Can you work these out from the drawing? Everything is in mm from the part's minimum corner. A direction names the side the tool comes from. Round coordinates to 2 decimals unless told otherwise and drop trailing zeros. Order: outer loops, then holes, each group sorted by start corner. A loop starts at its lowest first (then second) coordinate and runs counter-clockwise, first axis right, second up. Notation, with made-up numbers: M 38.25,47 L 89.25,47 A27 ccw 89.25,75 Z; hole C -30,39.5 d7. An arc over 180 degrees is marked long. Write item = value, one per line. Start each with the question number.
Item 1: For the marked faces 4 and 5, which set-ups out of +Z, -Z, +X, -X, +Y, -Y let a thin tool reach every point of the face, with its end or its side?
Item 2: I want a section at C-C, the plane z = 4.75. List the corners of the cut face in (x, y) for me (3 decimals), plus the area to 3 significant figures.
Item 3: I want a section at B-B, the plane x = 14. List the corners of the cut face in (y, z) for me.
Item 4: I'm going to push a flat-ended pin straight in: P1, Ø3, axis at x = 3.855, y = 23.32, coming from the -Z side. Where does the tip first touch, or does it pass through?
Item 5: I want a section at A-A, the plane y = 31.5. List the corners of the cut face in (x, z) for me (3 decimals), plus the area to 3 significant figures.
Item 6: I want a section at D-D, the plane y = 23.32. List the corners of the cut face in (x, z) for me (3 decimals).
Item 7: Please list where these lines run through material, in increasing order: L1, parallel to X at y = 23.32, z = 5.25 (3 decimals); L2, parallel to Y at x = 12, z = 1.75; L3, parallel to Y at x = 25, z = 2.25.
Item 8: We'd pull the mould along Y, two halves only. Please class the marked faces 1, 2 and 3: pulls with the +Y half, pulls with the -Y half, needs draft (parallel to the pull), parting line crosses it, or undercut.
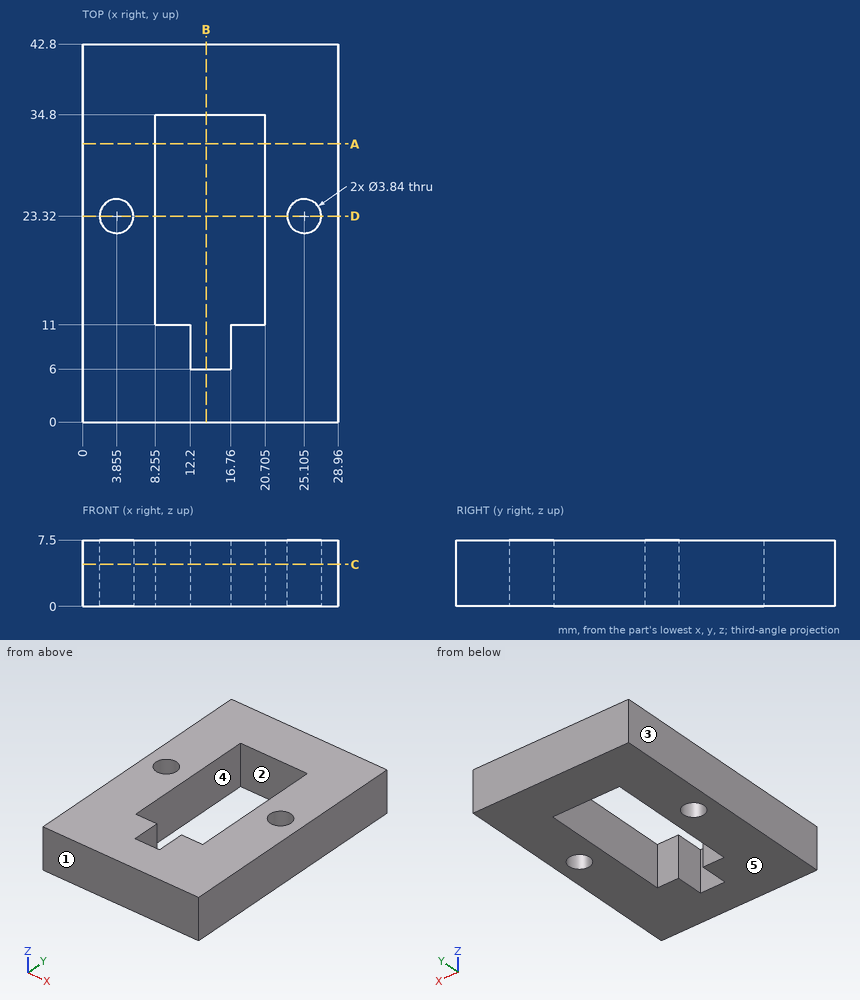
Filled in:
q1.face_4 = +Z, -Z
q1.face_5 = -Z, +X, -X, +Y, -Y
q2.outline = M 0,0 L 28.96,0 L 28.96,42.8 L 0,42.8 Z; hole C 3.855,23.32 d3.84; hole M 8.255,11 L 12.2,11 L 12.2,6 L 16.76,6 L 16.76,11 L 20.705,11 L 20.705,34.8 L 8.255,34.8 Z; hole C 25.105,23.32 d3.84
q2.area = 897 mm^2
q3.outline = M 0,0 L 6,0 L 6,7.5 L 0,7.5 Z; M 34.8,0 L 42.8,0 L 42.8,7.5 L 34.8,7.5 Z
q4.P1 = through
q5.outline = M 0,0 L 8.255,0 L 8.255,7.5 L 0,7.5 Z; M 20.705,0 L 28.96,0 L 28.96,7.5 L 20.705,7.5 Z
q5.area = 124 mm^2
q6.outline = M 0,0 L 1.935,0 L 1.935,7.5 L 0,7.5 Z; M 5.775,0 L 8.255,0 L 8.255,7.5 L 5.775,7.5 Z; M 20.705,0 L 23.185,0 L 23.185,7.5 L 20.705,7.5 Z; M 27.025,0 L 28.96,0 L 28.96,7.5 L 27.025,7.5 Z
q7.L1 = 0 to 1.935, 5.775 to 8.255, 20.705 to 23.185, 27.025 to 28.96
q7.L2 = 0 to 11, 34.8 to 42.8
q7.L3 = 0 to 21.4, 25.24 to 42.8
q8.face_1 = pulls with the -Y half
q8.face_2 = undercut
q8.face_3 = needs draft
